```python
from build123d import *

# Parameters (mm, degrees)
CROQUIS2_W              = 45
CROQUIS2_H              = 45
SALIENTE_EXTRUIR3_DEPTH = 1000
CROQUIS12_W             = 41
CROQUIS12_H             = 41
CORTAR_EXTRUIR8_DEPTH   = 1003.022953829
CROQUIS13_R             = 7
CORTAR_EXTRUIR9_DEPTH   = 1.6
CROQUIS15_R             = 7
CORTAR_EXTRUIR11_DEPTH  = 1003.022953829


with BuildPart() as part:
    # Croquis2 → Saliente-Extruir3 (new body)
    with BuildSketch(Plane.XY):
        with Locations((22.5, 22.5)):
            Rectangle(CROQUIS2_W, CROQUIS2_H)
    extrude(amount=SALIENTE_EXTRUIR3_DEPTH)

    # Croquis12 → Cortar-Extruir8 (cut, through all)
    with BuildSketch(Plane(origin=(0, 0, 0), x_dir=(-1, 0, 0), z_dir=(0, 0, -1))):
        with Locations((-22.5, 22.5)):
            Rectangle(CROQUIS12_W, CROQUIS12_H)
    extrude(amount=-CORTAR_EXTRUIR8_DEPTH, mode=Mode.SUBTRACT)

    # Croquis13 → Cortar-Extruir9 (cut)
    with BuildSketch(Plane.XZ):
        with Locations((22.5, 980)):
            Circle(CROQUIS13_R)
        with Locations((22.5, 940)):
            Circle(CROQUIS13_R)
        with Locations((22.5, 20)):
            Circle(CROQUIS13_R)
        with Locations((22.5, 60)):
            Circle(CROQUIS13_R)
    extrude(amount=-CORTAR_EXTRUIR9_DEPTH, mode=Mode.SUBTRACT)

    # Croquis15 → Cortar-Extruir11 (cut, through all)
    with BuildSketch(Plane.XZ):
        with Locations((21, 500)):
            Circle(CROQUIS15_R)
    extrude(amount=-CORTAR_EXTRUIR11_DEPTH, mode=Mode.SUBTRACT)


solid = part.part
```
Can you work these out from the model? Positions are in its coordinate system, mm. A direction names the side the tool comes from. Coordinates: 2 decimals unless noted, no trailing zeros. Loops run counter-clockwise (first coordinate to the right, second up) from the corner with the lowest first, then second, coordinate; pieces in that order, holes last. Notation, with made-up numbers: (-25.5, 81) - (-6.5, 81) arc R23 cw to (-6.5, 105) - close; hole circle Ø8 at (-17, -6.75). An arc over 180 degrees is marked (long way). Use a Markdown table: item, result.
Item 1: I want a section at B-B on y = 26.5. Please give me the cut outline in (x, z).
Numbers:
| item | result |
|---|---|
| outline | (0, 0) - (2, 0) - (2, 1000) - (0, 1000) - close; (43, 0) - (45, 0) - (45, 1000) - (43, 1000) - close |
Item 2: We'd pull the mould along X, two halves only. Please class faces 1 (the face through (23, 43, 493)), 2 (the face through (17, 45, 493)), 3 (the face through (0, 22, 493)): released by +X, released by -X, zero draft, split by the parting line, or undercut.
Numbers:
| item | result |
|---|---|
| face 1 | undercut |
| face 2 | zero draft |
| face 3 | released by -X |
Item 3: For faces 4 (the face through (21, 1, 1000)), 5 (the face through (23, 2, 493)), which set-ups out of +Z, -Z, +X, -X, +Y, -Y let a thin tool reach every point of the face, with its end or its side?
Numbers:
| item | result |
|---|---|
| face 4 | +Z, +X, -X, +Y, -Y |
| face 5 | +Z, -Z |
Item 4: I want a section at A-A on z = 909.5. Please give me the cut outline in (x, y).
Numbers:
| item | result |
|---|---|
| outline | (0, 0) - (45, 0) - (45, 45) - (0, 45) - close; hole (2, 2) - (43, 2) - (43, 43) - (2, 43) - close |
Item 5: Will these pins go through, and if not, where does the flat tip stop? pin 1 (18 mm diameter, centred on x = 21, z = 500, fed in from +Y); pin 2 (4 mm diameter, centred on x = 24.5, z = 941.5, fed in from -Y); pin 3 (6 mm diameter, centred on x = 23.5, y = 38, fed in from -Z).
Numbers:
| item | result |
|---|---|
| pin 1 | stops at y = 45 |
| pin 2 | stops at y = 1.6 |
| pin 3 | passes through |
Item 6: If I drill on probe 1 along Z at (x, y) = (22.5, 0.95); probe 2 along Y at (x, z) = (25, 48); probe 3 along Z at (x, y) = (21, 0.65), over which ranges is the centre line in solid material (lowest first)? Write a range as from..to.
Numbers:
| item | result |
|---|---|
| probe 1 | z = 0..13, 27..53, 67..493.16, 506.84..933, 947..973, 987..1000 |
| probe 2 | y = 0..2, 43..45 |
| probe 3 | z = 0..13.16, 26.84..53.16, 66.84..493, 507..933.16, 946.84..973.16, 986.84..1000 |
